Check sheet for the modelled part. Datum: model origin and axes. Units: mm. A direction names the side the tool comes from. Round coordinates to 2 decimals unless told otherwise and drop trailing zeros. Loops run counter-clockwise (first coordinate to the right, second up) from the corner with the lowest first, then second, coordinate; pieces in that order, holes last. Notation, with made-up numbers: (75.25, 10) - (124.25, 10) arc R28 ccw to (124.25, 46) - close; hole circle Ø1 at (71.5, 45.25). An arc over 180 degrees is marked (long way). Return JSON: item names as keys, results as strings.
from build123d import *

# Parameters (mm, degrees)
F1_DEPTH = 63.5
F0_W     = 24.7741062101
F0_H     = 19.05
F2_DEPTH = 25.4
F3_DEPTH = 7.9375
F5_R     = 6.35


with BuildPart() as f1:
    # F0 (on Front) → F1 (new body, symmetric)
    with BuildSketch(Plane.XZ):
        Polygon((22.225, 12.3348908712), (-41.275, 12.3348908712), (-41.275, -12.3348908712), (41.275, -12.3348908712), (41.275, 12.3348908712), align=None)
    extrude(amount=F1_DEPTH, both=True)

    # F0 (on Front) → F2 (join, symmetric)
    with BuildSketch(Plane.XZ):
        with BuildLine():
            Line((22.225, 24.1141091288), (22.225, 12.3348908712))
            Line((22.225, 12.3348908712), (41.275, 12.3348908712))
            Line((41.275, 12.3348908712), (41.275, 24.1141091288))
            ThreePointArc((41.275, 24.1141091288), (45.9246798487, 35.3394292801), (57.15, 39.9891091288))
            Line((57.15, 39.9891091288), (60.325, 39.9891091288))
            Line((60.325, 39.9891091288), (60.325, 59.0391091288))
            Line((60.325, 59.0391091288), (57.15, 59.0391091288))
            ThreePointArc((57.15, 59.0391091288), (32.4542956671, 48.8098134617), (22.225, 24.1141091288))
        make_face()
        with Locations((72.7120531051, 49.5141091288)):
            Rectangle(F0_W, F0_H)
    extrude(amount=F2_DEPTH, both=True)

    # F0 (on Front) → F3 (join, symmetric)
    with BuildSketch(Plane.XZ):
        with BuildLine():
            add(Edge.make_bspline(
                [(-41.275, 12.3348908712), (-32.6056554914, 51.0892942548), (21.4900877327, 66.2850886583), (57.15, 59.0391091288)],
                knots=[0, 0, 0, 0, 108.9438599833, 108.9438599833, 108.9438599833, 108.9438599833], degree=3))
            Line((-41.275, 12.3348908712), (22.225, 12.3348908712))
            Line((22.225, 12.3348908712), (22.225, 24.1141091288))
            ThreePointArc((22.225, 24.1141091288), (32.4542956671, 48.8098134617), (57.15, 59.0391091288))
        make_face()
    extrude(amount=F3_DEPTH, both=True)

    # F0 (on Front) → F4 (revolve)
    with BuildSketch(Plane.XZ):
        Polygon((111.125, 63.8651091288), (85.0991062101, 63.8651091288), (85.725, 35.2901091288), (111.125, 35.2901091288), align=None)
    revolve(axis=Axis((85.4120531051, 0, 49.5776091288), (-0.0218982923, 0, 0.9997602036)))

    # F5
    f5_edges = [f1.edges().sort_by_distance(p)[0] for p in [
        (-41.275, -63.5, 0),
        (41.275, -63.5, 0),
        (41.275, 63.5, 0),
        (-41.275, 63.5, 0),
    ]]
    fillet(f5_edges, radius=F5_R)


solid = f1.part
Q1. Sectioned sample at B-B (y = 47). Enter the section's corners in (x, z) (3 decimals).
Answer key:
{"outline": "(-41.275, -12.335) - (41.275, -12.335) - (41.275, 12.335) - (-41.275, 12.335) - close"}
Q2. Draft check along Y on faces 1 (the face through (59, -2, 59.039)), 2 (the face through (39.464, 61.59, 0.173)), 3 (the face through (84.14, 0.07, 35.22)). Enter one of: released by +Y, released by -Y, zero draft, split by the parting line, or undercut.
Answer key:
{"face 1": "zero draft", "face 2": "released by +Y", "face 3": "undercut"}
Q3. Scan lines: probe 1 along Y at (x, z) = (70, 58); probe 2 along Z at (x, y) = (29.5, 54); probe 3 along Y at (x, z) = (-7, 31). Record each from-to range of solid material in increasing order. Write a range as [from, to].
Answer key:
{"probe 1": "y = [-25.4, 25.4]", "probe 2": "z = [-12.33, 12.33]", "probe 3": "y = [-7.94, 7.94]"}
Q4. Depth check by flat-ended pin: P1, Ø8, axis at x = 42.5, z = 1.5, coming from the +Y side; P2, Ø13, axis at y = 17.5, z = 18, coming from the -X side (3 decimals); P3, Ø1.5, axis at y = 9, z = 19, coming from the -X side (3 decimals); P4, Ø13, axis at x = 69, y = 0.5, coming from the -Z side. Enter the tip coordinate at first touch or a pass-through.
Answer key:
{"P1": "stops at y = 62.4", "P2": "stops at x = -41.275", "P3": "stops at x = 22.225", "P4": "stops at z = 34.27"}
Q5. Tool access check on faces 4 (the face through (59.5, -0.1, 39.989)), 5 (the face through (45.802, -0.356, 35.215)), 6 (the face through (84.169, 0.854, 63.817)), 7 (the face through (-2, 7.938, 34)), 8 (the face through (32.73, -16.79, 49.08)). Record the directions out of +Z, -Z, +X, -X, +Y, -Y that give a thin tool (end or side, any length) a straight path to the whole face; none if there is none.
Answer key:
{"face 4": "-Z", "face 5": "-Z, +Y, -Y", "face 6": "+Z, -X", "face 7": "+Z, -X, +Y", "face 8": "+Z, -X, -Y"}
Q6. Sectioned sample at A-A (z = 7). Enter the section's corners in (x, y) (3 decimals), plus the area to 3 significant figures.
Answer key:
{"outline": "(-41.275, -57.15) arc R6.35 ccw to (-34.925, -63.5) - (34.925, -63.5) arc R6.35 ccw to (41.275, -57.15) - (41.275, 57.15) arc R6.35 ccw to (34.925, 63.5) - (-34.925, 63.5) arc R6.35 ccw to (-41.275, 57.15) - close", "area": "10,400 mm²"}
